The model under review builds one solid part; all positions refer to its coordinate system, in mm. Face numbers are marked on the shaded views. A direction names the side the tool comes from. Round coordinates to 2 decimals unless told otherwise and drop trailing zeros. Order: outer loops, then holes, each group sorted by start corner. A loop starts at its lowest first (then second) coordinate and runs counter-clockwise, first axis right, second up.
1) To check wall thickness, follow L1, parallel to Z at x = 54, y = 1; L2, parallel to Y at x = 5.5, z = 2.6; L3, parallel to Y at x = 21, z = 2. State the ranges of each line that lie inside material, in increasing order.
2) Consider section B-B (x = 12.8). Give the boundary of the cut face in (y, z), then the cut area to 3 significant figures.
3) Consider section C-C (y = 27.5). Give the boundary of the cut face in (x, z), then the cut area to 3 significant figures.
4) Mouldability with a two-part tool opening along Y and no side actions: class the marked faces 6, 7, 8 and 9 as pulls with the +Y half, pulls with the -Y half, needs draft (parallel to the pull), parting line crosses it, or undercut.
5) Machinability: for the marked faces 1, 2, 3, 4 and 5, which of the approach directions +Z, -Z, +X, -X, +Y, -Y give a long, thin tool a straight path to every point of the face, cutting with its end or side? Answer none if there is none.
6) Clearance check with flat-ended pins moving along their axes: P1, Ø6.5, axis at x = -2, z = 2.5, coming from the +Y side; P2, Ø12, axis at y = 3, z = -4, coming from the -X side; P3, Ø3, axis at y = -3.5, z = 2, coming from the +X side; P4, Ø20.5, axis at x = 21, y = 21, coming from the +Z side. State where each tip first meets the part, or that it passes through.
7) Consider section A-A (x = 55). Give the boundary of the cut face in (y, z), then the cut area to 3 significant figures.
8) Consider section D-D (z = -6). Give the boundary of the cut face in (x, y).
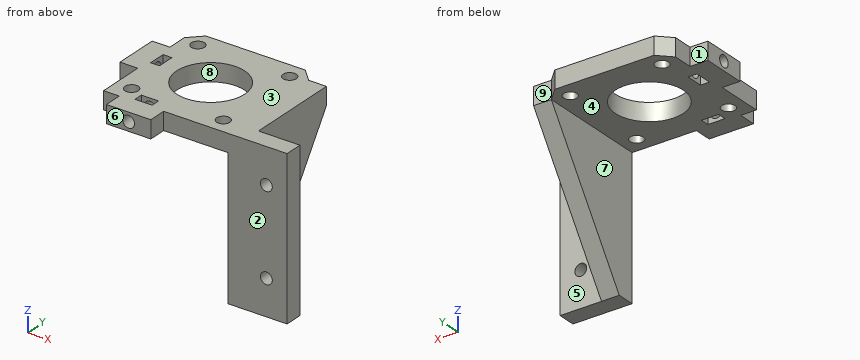
from build123d import *

# Parameters (mm, degrees)
ESQUISSE1_R             = 11.5
ESQUISSE1_R_2           = 2.25
ESQUISSE1_W             = 3
ESQUISSE1_H             = 5.8
ESQUISSE1_W_2           = 5.8
ESQUISSE1_H_2           = 3
BOSS_EXTRU_2_DEPTH      = 6
BOSS_EXTRU_4_DEPTH      = 6
ESQUISSE11_W            = 14
ESQUISSE11_H            = 53
ESQUISSE11_R            = 2
BOSS_EXTRU_5_DEPTH      = 6
ESQUISSE13_R            = 2
ENL_V_MAT_EXTRU_1_DEPTH = 14
ESQUISSE14_R            = 2
ENL_V_MAT_EXTRU_2_DEPTH = 14


with BuildPart() as part:
    # Esquisse1 → Boss.-Extru.2 (new body)
    with BuildSketch(Plane.XY):
        Polygon((0, 0), (0, 16), (-6, 16), (-6, 31), (0, 31), (0, 37.757359313), (4.242640687, 42), (37.757359313, 42), (42, 37.757359313), (42, 0), (20.3, 0), (20.3, -6), (5.3, -6), (5.3, 0), align=None)
        with Locations((21, 21)):
            Circle(ESQUISSE1_R, mode=Mode.SUBTRACT)
        with Locations((5.5, 36.5)):
            Circle(ESQUISSE1_R_2, mode=Mode.SUBTRACT)
        with Locations((36.5, 36.5)):
            Circle(ESQUISSE1_R_2, mode=Mode.SUBTRACT)
        with Locations((5.5, 5.5)):
            Circle(ESQUISSE1_R_2, mode=Mode.SUBTRACT)
        with Locations((36.5, 5.5)):
            Circle(ESQUISSE1_R_2, mode=Mode.SUBTRACT)
        with Locations((2.5, 23.5)):
            Rectangle(ESQUISSE1_W, ESQUISSE1_H, mode=Mode.SUBTRACT)
        with Locations((12.8, 2.5)):
            Rectangle(ESQUISSE1_W_2, ESQUISSE1_H_2, mode=Mode.SUBTRACT)
    extrude(amount=BOSS_EXTRU_2_DEPTH)

    # Esquisse9 → Boss.-Extru.4 (add)
    with BuildSketch(Plane(origin=(42, 0, 0), x_dir=(0, 0, -1), z_dir=(1, 0, 0))):
        Polygon((-6, 0), (47, 0), (47, 6), (0, 37.757359313), (-6, 37.757359313), align=None)
    extrude(amount=BOSS_EXTRU_4_DEPTH)

    # Esquisse11 → Boss.-Extru.5 (add)
    with BuildSketch(Plane.XZ):
        with Locations((55, -20.5)):
            Rectangle(ESQUISSE11_W, ESQUISSE11_H)
        with Locations((55, -35)):
            Circle(ESQUISSE11_R, mode=Mode.SUBTRACT)
        with Locations((55, -6)):
            Circle(ESQUISSE11_R, mode=Mode.SUBTRACT)
    extrude(amount=-BOSS_EXTRU_5_DEPTH)

    # Esquisse13 → Enlèv. mat.-Extru.1 (cut)
    with BuildSketch(Plane.ZY.offset(6)):
        with Locations((3, 23.5)):
            Circle(ESQUISSE13_R)
    extrude(amount=-ENL_V_MAT_EXTRU_1_DEPTH, mode=Mode.SUBTRACT)

    # Esquisse14 → Enlèv. mat.-Extru.2 (cut)
    with BuildSketch(Plane.XZ.offset(6)):
        with Locations((12.8, 3)):
            Circle(ESQUISSE14_R)
    extrude(amount=-ENL_V_MAT_EXTRU_2_DEPTH, mode=Mode.SUBTRACT)


solid = part.part
Answer below:
1. L1: z = -47 to -36.73, -33.27 to -7.73, -4.27 to 6
1. L2: y = -6 to 3.25, 7.75 to 21.54, 25.46 to 34.25, 38.75 to 42
1. L3: y = 0 to 9.5, 32.5 to 42
2. outline: (-6, 0) - (1, 0) - (1, 1) - (-6, 1) - close; (-6, 5) - (1, 5) - (1, 6) - (-6, 6) - close; (4, 0) - (12.94, 0) - (12.94, 6) - (4, 6) - (4, 5) - (8, 5) - (8, 1) - (4, 1) - close; (29.06, 0) - (42, 0) - (42, 6) - (29.06, 6) - close
2. area: 129 mm2
3. outline: (-6, 0) - (11.51, 0) - (11.51, 6) - (-6, 6) - close; (30.49, 0) - (42, 0) - (42, -15.18) - (48, -15.18) - (48, 6) - (30.49, 6) - close
3. area: 301 mm2
4. face 6: pulls with the -Y half
4. face 7: needs draft
4. face 8: undercut
4. face 9: pulls with the +Y half
5. face 1: +Z, -Z, -X, +Y
5. face 2: +Z, -Z, +X, -Y
5. face 3: +Z, +X, -X, +Y, -Y
5. face 4: -Z, -X, +Y, -Y
5. face 5: +Z, -Z, +X, +Y
6. P1: stops at y = 39.01
6. P2: stops at x = 0
6. P3: stops at x = 20.3
6. P4: passes through
7. outline: (0, -47) - (6, -47) - (6, -37) - (0, -37) - close; (0, -33) - (6, -33) - (6, -8) - (0, -8) - close; (0, -4) - (6, -4) - (6, 6) - (0, 6) - close
7. area: 270 mm2
8. outline: (42, 0) - (53, 0) - (53, 6) - (48, 6) - (48, 33.7) - (42, 33.7) - close; (57, 0) - (62, 0) - (62, 6) - (57, 6) - close
